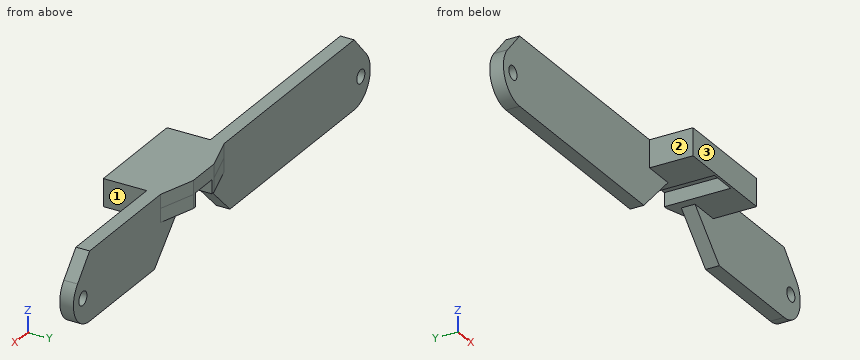
```python
from build123d import *
from OCP.BRepFilletAPI import BRepFilletAPI_MakeChamfer

# Parameters (mm, degrees)
SKETCH1_R           = 1.5
BOSS_EXTRUDE1_DEPTH = 3
CUT_EXTRUDE1_DEPTH  = 10
CUT_EXTRUDE3_START  = -3
SKETCH8_W           = 6
SKETCH8_H           = 3
CUT_EXTRUDE3_DEPTH  = 4
BOSS_EXTRUDE4_START = 2.5
BOSS_EXTRUDE4_DEPTH = 15
BOSS_EXTRUDE5_DEPTH = 3
BOSS_EXTRUDE6_START = 2.5
SKETCH11_W          = 8
SKETCH11_H          = 3
BOSS_EXTRUDE6_DEPTH = 15
CHAMFER1_SIZE       = 7.928987006
CHAMFER1_SIZE_2     = 2.5
SKETCH12_W          = 6
SKETCH12_H          = 0.5
BOSS_EXTRUDE7_DEPTH = 3
BOSS_EXTRUDE8_START = 6
BOSS_EXTRUDE8_DEPTH = 3
BOSS_EXTRUDE9_DEPTH = 3


with BuildPart() as part:
    # Sketch1 → Boss-Extrude1 (new body)
    with BuildSketch(Plane(origin=(0, 0, 0), x_dir=(1, 0, 0), z_dir=(0, 1, 0))):
        with BuildLine():
            Line((-49, 6), (49, 6))
            ThreePointArc((49, 6), (55, 0), (49, -6))
            Line((49, -6), (-49, -6))
            ThreePointArc((-49, -6), (-55, 0), (-49, 6))
        make_face()
        with Locations(Location((-51.5, 0, 0), (0, 0, 270))):
            Circle(SKETCH1_R, mode=Mode.SUBTRACT)
        with Locations(Location((51.5, 0, 0), (0, 0, 270))):
            Circle(SKETCH1_R, mode=Mode.SUBTRACT)
    extrude(amount=BOSS_EXTRUDE1_DEPTH)

    # Sketch2 → Cut-Extrude1 (cut)
    with BuildSketch(Plane(origin=(0, 3, 0), x_dir=(1, 0, 0), z_dir=(0, 1, 0))):
        Polygon((-9, 6), (0, -3), (22, -3), (31, 6), align=None)
    extrude(amount=-CUT_EXTRUDE1_DEPTH, mode=Mode.SUBTRACT)

    # Sketch8 → Cut-Extrude3 (cut)
    with BuildSketch(Plane.XY.offset(6).offset(CUT_EXTRUDE3_START)):
        with Locations((10.960071178, 1.5)):
            Rectangle(SKETCH8_W, SKETCH8_H)
    extrude(amount=CUT_EXTRUDE3_DEPTH, mode=Mode.SUBTRACT)


with BuildPart() as cut_extrude3_piece_1:
    # of the separate pieces the step leaves, piece 1, a body of its own (cut_extrude3_pieces)
    add(part.part.solids().sort_by_distance((-49, 0, -6))[0])

    # Sketch9 → Boss-Extrude4 (add)
    with BuildSketch(Plane(origin=(0, 3, 0), x_dir=(1, 0, 0), z_dir=(0, 1, 0)).offset(BOSS_EXTRUDE4_START)):
        Polygon((13.960071178, -6), (13.960071178, -3), (14.760071178, -3), (14.760071178, -6.8), (7.160071178, -6.8), (7.160071178, -3), (7.960071178, -3), (7.960071178, -6), align=None)
    extrude(amount=-BOSS_EXTRUDE4_DEPTH)



with BuildPart() as cut_extrude3_piece_2:
    # of the separate pieces the step leaves, piece 2, a body of its own (cut_extrude3_pieces)
    add(part.part.solids().sort_by_distance((49, 0, 6))[0])


with BuildPart() as cut_extrude3_piece_1_1:
    add(cut_extrude3_piece_1.part)

    add(cut_extrude3_piece_2.part)  # Boss-Extrude5 merges Cut-Extrude3 piece 2
    # Sketch10 → Boss-Extrude5 (add)
    with BuildSketch(Plane(origin=(0, 0, 0), x_dir=(1, 0, 0), z_dir=(0, 1, 0))):
        Polygon((22, -3), (16, -3), (25, 6), (31, 6), align=None)
        Polygon((0, -3), (6, -3), (-3, 6), (-9, 6), align=None)
    extrude(amount=BOSS_EXTRUDE5_DEPTH)

    # Sketch11 → Boss-Extrude6 (add)
    with BuildSketch(Plane(origin=(0, 3, 0), x_dir=(1, 0, 0), z_dir=(0, 1, 0)).offset(BOSS_EXTRUDE6_START)):
        with Locations((3.160071178, -4.5)):
            Rectangle(SKETCH11_W, SKETCH11_H)
        Polygon((16, -3), (14.760071178, -3), (14.760071178, -6), (22.760071178, -6), (22.760071178, -3), align=None)
    extrude(amount=-BOSS_EXTRUDE6_DEPTH)

    # Chamfer1
    chamfer1_edges_1 = [cut_extrude3_piece_1_1.edges().sort_by_distance(p)[0] for p in [
        (-0.839928822, 5.5, 4.5),
    ]]
    chamfer1_side_1 = [cut_extrude3_piece_1_1.faces().sort_by_distance(p)[0] for p in [
        (-0.789928822, 5.5, 4.5),
    ]]
    chamfer1_edges_2 = [cut_extrude3_piece_1_1.edges().sort_by_distance(p)[0] for p in [
        (22.760071178, 5.5, 4.5),
    ]]
    chamfer1_side_2 = [cut_extrude3_piece_1_1.faces().sort_by_distance(p)[0] for p in [
        (22.760071178, 5.45, 4.5),
    ]]
    chamfer1 = BRepFilletAPI_MakeChamfer(cut_extrude3_piece_1_1.part.solid().wrapped)
    for e in chamfer1_edges_1:
        chamfer1.Add(CHAMFER1_SIZE - 0.0001, CHAMFER1_SIZE_2 - 0.0001, e.wrapped, chamfer1_side_1[0].wrapped)
    for e in chamfer1_edges_2:
        chamfer1.Add(CHAMFER1_SIZE_2 - 0.0001, CHAMFER1_SIZE - 0.0001, e.wrapped, chamfer1_side_2[0].wrapped)
    add(Compound.cast(chamfer1.Shape()), mode=Mode.REPLACE)  # a hair under: the kernel refuses the full size

    # Sketch12 → Boss-Extrude7 (add)
    with BuildSketch(Plane(origin=(0, 0, 6), x_dir=(-1, 0, 0), z_dir=(0, 0, -1))):
        with Locations((-10.960071178, -9.25)):
            Rectangle(SKETCH12_W, SKETCH12_H)
    extrude(amount=BOSS_EXTRUDE7_DEPTH)

    # Sketch13 → Boss-Extrude8 (add)
    with BuildSketch(Plane.XY.offset(BOSS_EXTRUDE8_START)):
        Polygon((7.160071178, 5.5), (-0.839928822, 3), (-49, 3), (-49, 0), (-0.839928822, 0), (-0.839928822, -9.5), (7.160071178, -9.5), (14.760071178, -9.5), (22.760071178, -9.5), (22.760071178, 0), (49, 0), (49, 3), (22.760071178, 3), (14.831084172, 5.5), (14.760071178, 5.5), align=None)
    extrude(amount=BOSS_EXTRUDE8_DEPTH)

    # Sketch14 → Boss-Extrude9 (add)
    with BuildSketch(Plane(origin=(0, 3, 0), x_dir=(1, 0, 0), z_dir=(0, 1, 0))):
        with BuildLine():
            Line((-49, -9), (-53.472135955, -4))
            ThreePointArc((-53.472135955, -4), (-51.449489743, -5.477225575), (-49, -6))
            Line((-49, -6), (-49, -9))
        make_face()
        with BuildLine():
            Line((49, -9), (53.472135955, -4))
            ThreePointArc((53.472135955, -4), (51.449489743, -5.477225575), (49, -6))
            Line((49, -6), (49, -9))
        make_face()
    extrude(amount=-BOSS_EXTRUDE9_DEPTH)


solid = cut_extrude3_piece_1_1.part
```
The listing builds one solid part. Answer for the finished solid, in the listing's coordinates (mm). Face numbers are marked on the shaded views. A direction names the side the tool comes from. Give positions to 0.01 mm unless a question says otherwise; leave off trailing zeros. Order: outer loops, then holes, each group sorted by start corner. A loop starts at its lowest first (then second) coordinate and runs counter-clockwise, first axis right, second up. Notation, with made-up numbers: (63.25, -33.75) -> (112.25, -33.75) arc R19 ccw to (112.25, -1.75) -> close; hole circle Ø4 at (-24, 69). An arc over 180 degrees is marked (long way). Answer as a JSON object with one key per item and string values. Group by question number.
Item 1: The part is cut by section C-C on z = -5. Write down the section's boundary in (x, y), and give its area (3 significant figures).
Item 2: The part is cut by section B-B on y = -5.75. Write down the section's boundary in (x, z), and give its area (3 significant figures).
Item 3: The part is cut by section A-A on z = 0. Write down the section's boundary in (x, y), and give its area (3 significant figures).
Item 4: Consider L1, parallel to X at y = 0.95, z = 0; L2, parallel to X at y = 2.75, z = 0.5; L3, parallel to Y at x = -19, z = 0.5. Determine where each line is inside the solid, lowest interval first. Write a range as from..to.
Item 5: The part is cut by section D-D on x = -51.5. Write down the section's boundary in (y, z).
Item 6: A tool of negligible diameter and unlimited length cuts with its end or side. For the marked faces 1, 2 and 3, from which of +Z, -Z, +X, -X, +Y, -Y can it reach the whole face along a straight path? Write none if from no direction.
Item 7: Flat-ended cylindrical pins translate along their axes: pin 1 (3 mm diameter, centred on x = -7.5, z = 3, fed in from -Y); pin 2 (1.5 mm diameter, centred on y = -4, z = 4, fed in from +X); pin 3 (4 mm diameter, centred on x = -5, z = 3.5, fed in from +Y); pin 4 (0.8 mm diameter, centred on x = 4, y = 5, fed in from +Z). Find the tip coordinate at first contact, or state that the pin passes through.
Result set:
{
 "1": {"outline": "(-52.32, 0) -> (-2, 0) -> (-2, 3) -> (-52.32, 3) -> close; (24, 0) -> (52.32, 0) -> (52.32, 3) -> (24, 3) -> close", "area": "236 mm²"},
 "2": {"outline": "(-0.84, 3) -> (7.96, 3) -> (7.96, 6) -> (13.96, 6) -> (13.96, 3) -> (22.76, 3) -> (22.76, 9) -> (-0.84, 9) -> close", "area": "124 mm²"},
 "3": {"outline": "(-55, 0) -> (-53, 0) -> (-53, 3) -> (-55, 3) -> close; (-50, 0) -> (3, 0) -> (3, 3) -> (-50, 3) -> close; (19, 0) -> (50, 0) -> (50, 3) -> (19, 3) -> close; (53, 0) -> (55, 0) -> (55, 3) -> (53, 3) -> close", "area": "264 mm²"},
 "4": {"L1": "-55..-53, -50..3, 19..50, 53..55", "L2": "-54.98..-52.91, -50.09..3.5, 18.5..50.09, 52.91..54.98", "L3": "0..3"},
 "5": {"outline": "(0, -5.45) -> (3, -5.45) -> (3, -1.5) -> (0, -1.5) -> close; (0, 1.5) -> (3, 1.5) -> (3, 6.2) -> (0, 6.2) -> close"},
 "6": {"face 1": "+Z, -Z, +X, -Y", "face 2": "+Z, -Z, -X, -Y", "face 3": "+Z, -Z, +X, -X, -Y"},
 "7": {"pin 1": "y = 0", "pin 2": "x = 22.76", "pin 3": "y = 3", "pin 4": "through"}
}
